Check sheet for the modelled part. Datum: model origin and axes. Units: mm. Coordinates: 2 decimals unless noted, no trailing zeros. Loops run counter-clockwise (first coordinate to the right, second up) from the corner with the lowest first, then second, coordinate; pieces in that order, holes last. Notation, with made-up numbers: (70.5, -12.75) - (126.5, -12.75) arc R14 cw to (126.5, -2.75) - close; hole circle Ø8 at (61, -10). An arc over 180 degrees is marked (long way). Answer as a JSON object with one key per item and string values. Group by question number.
Autodesk Inventor part; units mm, degrees
ref_plane "YZ Plane" through (0, 0, 0) normal (1, 0, 0) x (0, 1, 0)
ref_plane "XZ Plane" through (0, 0, 0) normal (0, 1, 0) x (-1, 0, 0)
ref_plane "XY Plane" through (0, 0, 0) normal (0, 0, 1) x (1, 0, 0)
sketch "Sketch3" plane through (0, 0, 0) normal (0, 0, 1) x (1, 0, 0)
  circle A0 centre (0, 0) radius 5
  dimension "d0" = 10
extrude "Extrusion1" add sketch "Sketch3" against normal blind 100
sketch "Sketch4" plane through (0, 0, 0) normal (0, 1, 0) x (-1, 0, 0)
  circle A0 centre (0, -10) radius 1.5
  line L0 (5, 0) -> (-5, 0)
  point P0 (0, 0)
  dimension "d3" = 3
  dimension "d11" = 10
hole "Hole1" at (0, 0, -10) direction (0, -1, 0) diameter 3 end through all both
sketch "Sketch14" plane through (0, 0, 0) normal (0, 1, 0) x (-1, 0, 0)
  line L0 (-5, 0) -> (-5, -100)
  line L1 (-5, -61) -> (-4.6, -61)
  line L2 (-4.6, -61) -> (-4.6, -60)
  line L3 (-4.6, -60) -> (-5, -60)
  line L4 (-5, -60) -> (-5, -61)
  line L5 (5, 0) -> (-5, 0)
  line L6 (0, -120) -> (0, 20)
  point P0 (0, 0)
  dimension "d22" = 60
  dimension "d23" = 0.4
  dimension "d24" = 1
revolve "Revolution2" cut sketch "Sketch14" angle 360 about axis through (0, 0, 0) along (0, 0, -1)
equation "\"BendRadius\" = Thickness"
equation "\"BendReliefWidth\" = Thickness"
equation "\"BendReliefDepth\" = 0.5 * Thickness"
equation "\"CornerReliefSize\" = 4 * Thickness"
equation "\"MinimumRemnant\" = 2 * Thickness"
equation "\"TransitionRadius\" = BendRadius"
equation "\"JacobiRadiusSize\" = BendRadius"
equation "\"GapSize\" = Thickness"
properties part number "Shaft_piston"
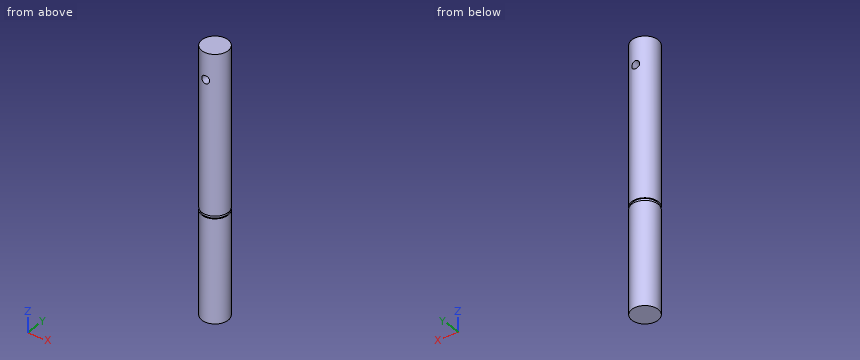
1. Sectioned sample at D-D on z = -34.5. Record the cut outline in (x, y).
2. Material ranges on line 1 (Z direction, x = 0, y = 1.25); line 2 (X direction, y = 2, z = -10); line 3 (X direction, y = 2.25, z = -10), recorded low to high.
3. Gauge pin test, flat ends, axial feed: pin 1 (3.5 mm diameter, centred on x = 0, z = -10, fed in from +Y); pin 2 (2 mm diameter, centred on x = -3, z = -31, fed in from +Y). Record the tip position at first contact, or that the pin passes through.
4. Sectioned sample at C-C on z = -10. Record the cut outline in (x, y).
5. Sectioned sample at A-A on x = 0. Record the cut outline in (y, z), plus the area to 3 significant figures.
6. Sectioned sample at B-B on y = -3. Record the cut outline in (x, z).
Answers follow:
{
 "1": {"outline": "circle Ø10 at (0, 0)"},
 "2": {"line 1": "z = -100 to -11.5, -8.5 to 0", "line 2": "x = -4.58 to -1.5, 1.5 to 4.58", "line 3": "x = -4.47 to -1.5, 1.5 to 4.47"},
 "3": {"pin 1": "stops at y = 5", "pin 2": "stops at y = 4.58"},
 "4": {"outline": "(-1.5, -4.77) - (-1.5, 4.77) arc R5 ccw to start; (1.5, -4.77) arc R5 ccw to (1.5, 4.77) - close"},
 "5": {"outline": "(-5, -100) - (5, -100) - (5, -61) - (4.6, -61) - (4.6, -60) - (5, -60) - (5, -11.5) - (-5, -11.5) - (-5, -60) - (-4.6, -60) - (-4.6, -61) - (-5, -61) - close; (-5, -8.5) - (5, -8.5) - (5, 0) - (-5, 0) - close", "area": "969 mm^2"},
 "6": {"outline": "(-4, -100) - (4, -100) - (4, -61) - (3.49, -61) - (3.49, -60) - (4, -60) - (4, 0) - (-4, 0) - (-4, -60) - (-3.49, -60) - (-3.49, -61) - (-4, -61) - close; hole circle Ø3 at (0, -10)"}
}
